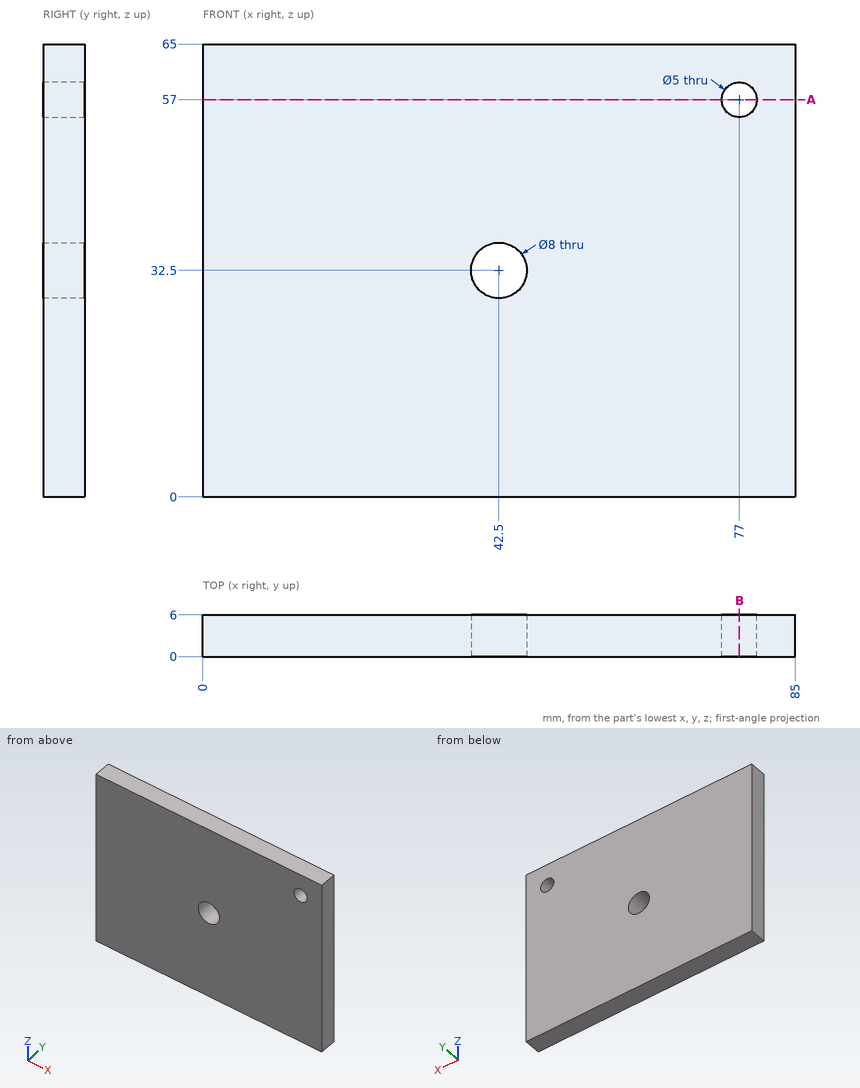
Can you work these out from the drawing? Everything is in mm from the part's minimum corner. Round coordinates to 2 decimals unless told otherwise and drop trailing zeros. Loops run counter-clockwise (first coordinate to the right, second up) from the corner with the lowest first, then second, coordinate; pieces in that order, holes last. Notation, with made-up numbers: (-16.5, 64) -> (18.5, 64) arc R27 ccw to (18.5, 81) -> close; hole circle Ø8 at (-36.5, 43.25). An arc over 180 degrees is marked (long way). Use CSV: the item, a comma, the result in double quotes.
(1) Suppose I cut it at A-A on z = 57. Write out the boundary of the cut face in (x, y).
Return value:
outline,"(0, 0) -> (74.5, 0) -> (74.5, 6) -> (0, 6) -> close; (79.5, 0) -> (85, 0) -> (85, 6) -> (79.5, 6) -> close"
(2) Will this pin go through, and if not, where does the flat tip stop? pin 1 Ø3 at (x, z) = (77, 57) entering from -Y.
Return value:
pin 1,"passes through"
(3) If I drill on probe 1 along X at (y, z) = (1.9, 57); probe 2 along X at (y, z) = (1, 32.5); probe 3 along Z at (x, y) = (43, 2.6), over which ranges is the centre line in solid material (lowest first)? Write a range as [from, to].
Return value:
probe 1,"x = [0, 74.5], [79.5, 85]"
probe 2,"x = [0, 38.5], [46.5, 85]"
probe 3,"z = [0, 28.53], [36.47, 65]"
(4) Suppose I cut it at B-B on x = 77. Write out the boundary of the cut face in (y, z), plus the area to 3 significant figures.
Return value:
outline,"(0, 0) -> (6, 0) -> (6, 54.5) -> (0, 54.5) -> close; (0, 59.5) -> (6, 59.5) -> (6, 65) -> (0, 65) -> close"
area,"360 mm²"
